Could you check a few things on this model? Use its own coordinates, in mm. Give positions to 0.01 mm unless a question says otherwise; leave off trailing zeros. Write each loop counter-clockwise with the first axis right and the second up, starting at its lowest first coordinate (ties: lowest second). Pieces come first, ordered by that corner, then holes. Notation, with made-up numbers: M -21.5,40 L 26.5,40 A6 cw 26.5,45 Z; hole C 54.25,61.25 d1. An arc over 180 degrees is marked long. Answer as CSV lines item,"result". Start each with the question number.
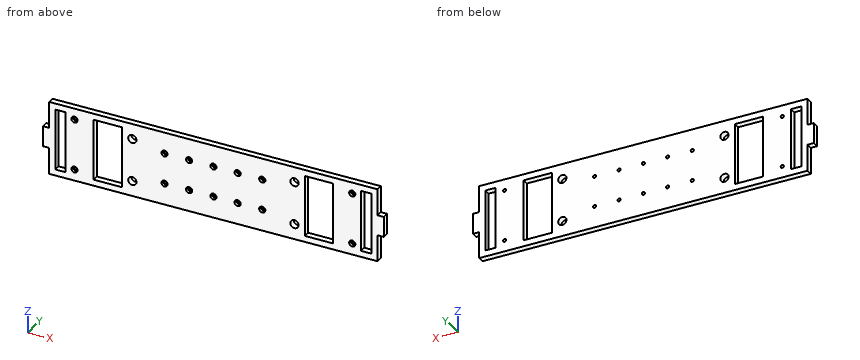
from build123d import *

# Parameters (mm, degrees)
BOSS_EXTRU_1_DEPTH      = 6
ESQUISSE2_R             = 1.5
ENL_V_MAT_EXTRU_1_DEPTH = 169.988165266
ESQUISSE3_R             = 3
ENL_V_MAT_EXTRU_2_DEPTH = 3
ESQUISSE4_R             = 4
ENL_V_MAT_EXTRU_3_DEPTH = 169.988165266
ESQUISSE5_W             = 27.5
ESQUISSE5_H             = 60
ENL_V_MAT_EXTRU_4_DEPTH = 169.988165266
ESQUISSE6_R             = 1.5
ENL_V_MAT_EXTRU_5_DEPTH = 169.988165266
ESQUISSE7_W             = 10
ESQUISSE7_H             = 60
ENL_V_MAT_EXTRU_6_DEPTH = 169.988165266
ESQUISSE8_R             = 3
ENL_V_MAT_EXTRU_7_DEPTH = 3


with BuildPart() as part:
    # Esquisse1 → Boss.-Extru.1 (new body)
    with BuildSketch(Plane(origin=(0, 0, 0), x_dir=(1, 0, 0), z_dir=(0, 1, 0))):
        Polygon((-159, -36), (-159, -10), (-165, -10), (-165, 10), (-159, 10), (-159, 36), (159, 36), (159, 10), (165, 10), (165, -10), (159, -10), (159, -36), align=None)
    extrude(amount=BOSS_EXTRU_1_DEPTH)

    # Esquisse2 → Enlèv. mat.-Extru.1 (cut, through all)
    with BuildSketch(Plane.XZ):
        with Locations(Location((-47.35, 15, 0), (0, 0, 270))):
            Circle(ESQUISSE2_R)
        with Locations(Location((-23.5, 15, 0), (0, 0, 270))):
            Circle(ESQUISSE2_R)
        with Locations(Location((23.5, 15, 0), (0, 0, 90))):
            Circle(ESQUISSE2_R)
        with Locations(Location((47.35, 15, 0), (0, 0, 90))):
            Circle(ESQUISSE2_R)
        with Locations(Location((47.35, -15, 0), (0, 0, 270))):
            Circle(ESQUISSE2_R)
        with Locations(Location((23.5, -15, 0), (0, 0, 270))):
            Circle(ESQUISSE2_R)
        with Locations(Location((-23.5, -15, 0), (0, 0, 90))):
            Circle(ESQUISSE2_R)
        with Locations(Location((-47.35, -15, 0), (0, 0, 90))):
            Circle(ESQUISSE2_R)
        with Locations(Location((0, 15, 0), (0, 0, 270))):
            Circle(ESQUISSE2_R)
        with Locations(Location((0, -15, 0), (0, 0, 90))):
            Circle(ESQUISSE2_R)
    extrude(amount=-ENL_V_MAT_EXTRU_1_DEPTH, mode=Mode.SUBTRACT)

    # Esquisse3 → Enlèv. mat.-Extru.2 (cut)
    with BuildSketch(Plane(origin=(0, 0, 0), x_dir=(-1, 0, 0), z_dir=(0, -1, 0))):
        with Locations(Location((47.35, -15, 0), (0, 0, 90))):
            Circle(ESQUISSE3_R)
        with Locations(Location((23.5, -15, 0), (0, 0, 90))):
            Circle(ESQUISSE3_R)
        with Locations(Location((0, -15, 0), (0, 0, 90))):
            Circle(ESQUISSE3_R)
        with Locations(Location((0, 15, 0), (0, 0, 270))):
            Circle(ESQUISSE3_R)
        with Locations(Location((23.5, 15, 0), (0, 0, 270))):
            Circle(ESQUISSE3_R)
        with Locations(Location((47.35, 15, 0), (0, 0, 270))):
            Circle(ESQUISSE3_R)
        with Locations(Location((-47.35, 15, 0), (0, 0, 90))):
            Circle(ESQUISSE3_R)
        with Locations(Location((-23.5, 15, 0), (0, 0, 90))):
            Circle(ESQUISSE3_R)
        with Locations(Location((-23.5, -15, 0), (0, 0, 270))):
            Circle(ESQUISSE3_R)
        with Locations(Location((-47.35, -15, 0), (0, 0, 270))):
            Circle(ESQUISSE3_R)
    extrude(amount=-ENL_V_MAT_EXTRU_2_DEPTH, mode=Mode.SUBTRACT)

    # Esquisse4 → Enlèv. mat.-Extru.3 (cut, through all)
    with BuildSketch(Plane(origin=(0, 0, 0), x_dir=(-1, 0, 0), z_dir=(0, -1, 0))):
        with Locations(Location((78.5, -21, 0), (0, 0, 90))):
            Circle(ESQUISSE4_R)
        with Locations(Location((-78.5, -21, 0), (0, 0, 270))):
            Circle(ESQUISSE4_R)
        with Locations(Location((78.5, 21, 0), (0, 0, 270))):
            Circle(ESQUISSE4_R)
        with Locations(Location((-78.5, 21, 0), (0, 0, 90))):
            Circle(ESQUISSE4_R)
    extrude(amount=-ENL_V_MAT_EXTRU_3_DEPTH, mode=Mode.SUBTRACT)

    # Esquisse5 → Enlèv. mat.-Extru.4 (cut, through all)
    with BuildSketch(Plane(origin=(0, 0, 0), x_dir=(-1, 0, 0), z_dir=(0, -1, 0))):
        with Locations((102.25, 0)):
            Rectangle(ESQUISSE5_W, ESQUISSE5_H)
        with Locations((-102.25, 0)):
            Rectangle(ESQUISSE5_W, ESQUISSE5_H)
    extrude(amount=-ENL_V_MAT_EXTRU_4_DEPTH, mode=Mode.SUBTRACT)

    # Esquisse6 → Enlèv. mat.-Extru.5 (cut, through all)
    with BuildSketch(Plane(origin=(0, 0, 0), x_dir=(-1, 0, 0), z_dir=(0, -1, 0))):
        with Locations(Location((134.5, -25, 0), (0, 0, 90))):
            Circle(ESQUISSE6_R)
        with Locations(Location((-134.5, -25, 0), (0, 0, 270))):
            Circle(ESQUISSE6_R)
        with Locations(Location((-134.5, 25, 0), (0, 0, 90))):
            Circle(ESQUISSE6_R)
        with Locations(Location((134.5, 25, 0), (0, 0, 270))):
            Circle(ESQUISSE6_R)
    extrude(amount=-ENL_V_MAT_EXTRU_5_DEPTH, mode=Mode.SUBTRACT)

    # Esquisse7 → Enlèv. mat.-Extru.6 (cut, through all)
    with BuildSketch(Plane(origin=(0, 0, 0), x_dir=(-1, 0, 0), z_dir=(0, -1, 0))):
        with Locations((148, 0)):
            Rectangle(ESQUISSE7_W, ESQUISSE7_H)
        with Locations((-148, 0)):
            Rectangle(ESQUISSE7_W, ESQUISSE7_H)
    extrude(amount=-ENL_V_MAT_EXTRU_6_DEPTH, mode=Mode.SUBTRACT)

    # Esquisse8 → Enlèv. mat.-Extru.7 (cut)
    with BuildSketch(Plane.XZ):
        with Locations(Location((-134.5, 25, 0), (0, 0, 270))):
            Circle(ESQUISSE8_R)
        with Locations(Location((-134.5, -25, 0), (0, 0, 270))):
            Circle(ESQUISSE8_R)
        with Locations(Location((134.5, -25, 0), (0, 0, 90))):
            Circle(ESQUISSE8_R)
        with Locations(Location((134.5, 25, 0), (0, 0, 90))):
            Circle(ESQUISSE8_R)
    extrude(amount=-ENL_V_MAT_EXTRU_7_DEPTH, mode=Mode.SUBTRACT)


solid = part.part
1. Please list where these lines run through material, in increasing order: line 1 (Z direction, x = -134.5, y = 0.8); line 2 (X direction, y = 0.65, z = -11); line 3 (X direction, y = 3.6, z = -1).
2. Imagine slicing it at B-B, the plane x = -78.5. Please give me the cut outline in (y, z).
3. Will these pins go through, and if not, where does the flat tip stop? P1, Ø3, axis at y = 4.5, z = 21, coming from the -X side; P2, Ø1.8, axis at x = 1.5, z = -15.5, coming from the -Y side; P3, Ø1.5, axis at y = 4, z = -15.5, coming from the +X side.
4. Imagine slicing it at C-C, the plane y = 1.2. State how many separate pieces and enclosed holes the cut face has, plus the area to 3 significant figures.
5. Imagine slicing it at A-A, the plane x = -112. Please give me the cut outline in (y, z), plus the area to 3 significant figures.
Solutions:
1,line 1,"-36 to -28, -22 to 22, 28 to 36"
1,line 2,"-159 to -153, -143 to -116, -88.5 to 88.5, 116 to 143, 153 to 159"
1,line 3,"-165 to -153, -143 to -116, -88.5 to 88.5, 116 to 143, 153 to 165"
2,outline,"M 0,-36 L 6,-36 L 6,-25 L 0,-25 Z; M 0,-17 L 6,-17 L 6,17 L 0,17 Z; M 0,25 L 6,25 L 6,36 L 0,36 Z"
3,P1,"x = -159"
3,P2,"y = 3"
3,P3,"x = 159"
4,separate pieces,"1"
4,enclosed holes,"22"
4,area,"18,000 mm²"
5,outline,"M 0,-36 L 6,-36 L 6,-30 L 0,-30 Z; M 0,30 L 6,30 L 6,36 L 0,36 Z"
5,area,"72.0 mm²"
